Can you work these out from the model? Positions are in its coordinate system, mm. Face numbers are marked on the shaded views. A direction names the side the tool comes from. Give positions to 0.01 mm unless a question says otherwise; leave off trailing zeros. Order: outer loops, then holes, each group sorted by start corner. A loop starts at its lowest first (then second) coordinate and runs counter-clockwise, first axis right, second up. Notation, with made-up numbers: (63, 44.5) -> (70, 44.5) arc R34 cw to (70, 81.5) -> close; hole circle Ø7 at (70, 57). An arc over 180 degrees is marked (long way). Answer as a JSON object with one key per item and string values.
```python
from build123d import *

# Parameters (mm, degrees)
SKETCH1_R           = 110
BOSS_EXTRUDE1_DEPTH = 12
SKETCH2_R           = 110
BOSS_EXTRUDE2_DEPTH = 55
SKETCH3_W           = 100
SKETCH3_H           = 100
BOSS_EXTRUDE3_DEPTH = 80
SKETCH4_R           = 30
BOSS_EXTRUDE4_DEPTH = 20
BOSS_EXTRUDE4_TAPER = 18
SHELL1_T            = -1
SKETCH6_W           = 98
SKETCH6_H           = 6.826689401
BOSS_EXTRUDE5_DEPTH = 100
SKETCH7_W           = 98
SKETCH7_H           = 74.173310599
BOSS_EXTRUDE6_DEPTH = 15
SKETCH8_W           = 98
SKETCH8_H           = 4.922598218
BOSS_EXTRUDE7_DEPTH = 83


with BuildPart() as part:
    # Sketch1 → Boss-Extrude1 (new body)
    with BuildSketch(Plane(origin=(0, 0, 0), x_dir=(1, 0, 0), z_dir=(0, 1, 0))):
        with Locations(Location((0, 0, 0), (0, 0, 270))):
            Circle(SKETCH1_R)
        with BuildLine():
            Line((-4.5, 8.309783391), (-4.5, 23.309783391))
            Line((-4.5, 23.309783391), (4.5, 23.309783391))
            Line((4.5, 23.309783391), (4.5, 8.309783391))
            ThreePointArc((4.5, 8.309783391), (9.45, 0), (4.5, -8.309783391))
            Line((4.5, -8.309783391), (4.5, -23.309783391))
            Line((4.5, -23.309783391), (-4.5, -23.309783391))
            Line((-4.5, -23.309783391), (-4.5, -8.309783391))
            ThreePointArc((-4.5, -8.309783391), (-9.45, 0), (-4.5, 8.309783391))
        make_face(mode=Mode.SUBTRACT)
    extrude(amount=BOSS_EXTRUDE1_DEPTH)

    # Sketch2 → Boss-Extrude2 (add)
    with BuildSketch(Plane(origin=(0, 12, 0), x_dir=(1, 0, 0), z_dir=(0, 1, 0))):
        with Locations(Location((0, 0, 0), (0, 0, 270))):
            Circle(SKETCH2_R)
    extrude(amount=BOSS_EXTRUDE2_DEPTH)

    # Sketch3 → Boss-Extrude3 (add)
    with BuildSketch(Plane(origin=(0, 67, 0), x_dir=(1, 0, 0), z_dir=(0, 1, 0))):
        Rectangle(SKETCH3_W, SKETCH3_H)
    extrude(amount=BOSS_EXTRUDE3_DEPTH)

    # Sketch4 → Boss-Extrude4 (add)
    with BuildSketch(Plane.XY.offset(50)):
        with Locations((0, 107)):
            Circle(SKETCH4_R)
    extrude(amount=BOSS_EXTRUDE4_DEPTH, taper=BOSS_EXTRUDE4_TAPER)

    # Shell1
    shell1_openings = [part.faces().sort_by_distance(p)[0] for p in [
        (0, 147, 0),
    ]]
    offset(amount=SHELL1_T, openings=shell1_openings, kind=Kind.INTERSECTION)

    # Sketch6 → Boss-Extrude5 (add)
    with BuildSketch(Plane.XY.offset(-49)):
        with Locations((0, 69.413344701)):
            Rectangle(SKETCH6_W, SKETCH6_H)
    extrude(amount=BOSS_EXTRUDE5_DEPTH)

    # Sketch7 → Boss-Extrude6 (add)
    with BuildSketch(Plane.XY.offset(-49)):
        with Locations((0, 109.913344701)):
            Rectangle(SKETCH7_W, SKETCH7_H)
    extrude(amount=BOSS_EXTRUDE6_DEPTH)

    # Sketch8 → Boss-Extrude7 (add)
    with BuildSketch(Plane.XY.offset(-34)):
        with Locations((0, 144.538700891)):
            Rectangle(SKETCH8_W, SKETCH8_H)
    extrude(amount=BOSS_EXTRUDE7_DEPTH)


solid = part.part
```
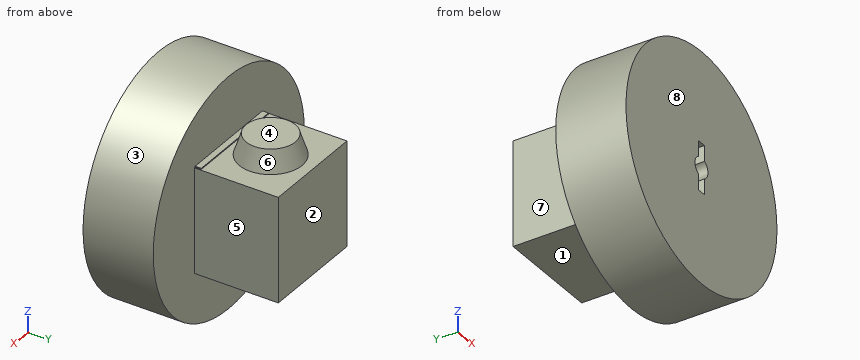
1. Will these pins go through, and if not, where does the flat tip stop? pin 1 Ø1.5 at (x, z) = (52, 52.5) entering from +Y; pin 2 Ø6 at (y, z) = (8, -17.5) entering from +X; pin 3 Ø23 at (x, y) = (-8.5, 106) entering from -Z; pin 4 Ø25 at (x, z) = (22, 22) entering from -Y.
Worked answers:
{"pin 1": "y = 67", "pin 2": "x = 109.04", "pin 3": "z = -50", "pin 4": "y = 0"}
2. Please list where these lines run through material, in increasing order: L1, parallel to Y at x = 48, z = -9.5; L2, parallel to Z at x = -45.5, y = 82; L3, parallel to Y at x = -87, z = -4.5.
Worked answers:
{"L1": "0 to 1, 66 to 72.83, 142.08 to 147", "L2": "-50 to -34, 49 to 50", "L3": "0 to 1, 66 to 67"}
3. If we section it at B-B on x = 0: Count the separate pieces of the cut face and the enclosed holes in it, then the cut area to 3 significant figures.
Worked answers:
{"separate pieces": "1", "enclosed holes": "2", "area": "2,880 mm²"}
4. If we section it at A-A on z = 0: Please give me the cut outline in (x, y), then the cut area to 3 significant figures.
Worked answers:
{"outline": "(-110, 0) -> (-9.45, 0) -> (-9.45, 12) -> (9.45, 12) -> (9.45, 0) -> (110, 0) -> (110, 67) -> (50, 67) -> (50, 147) -> (-50, 147) -> (-50, 67) -> (-110, 67) -> close; hole (-109, 1) -> (-10.45, 1) -> (-10.45, 13) -> (10.45, 13) -> (10.45, 1) -> (109, 1) -> (109, 66) -> (-109, 66) -> close; hole (-49, 72.83) -> (49, 72.83) -> (49, 142.08) -> (-49, 142.08) -> close", "area": "1,810 mm²"}
5. If we section it at C-C on y = 107: Please give me the cut outline in (x, z), then the cut area to 3 significant figures.
Worked answers:
{"outline": "(-50, -50) -> (50, -50) -> (50, 50) -> (30, 50) -> (23.5, 70) -> (-23.5, 70) -> (-30, 50) -> (-50, 50) -> close; hole (-49, -34) -> (49, -34) -> (49, 49) -> (29.27, 49) -> (22.78, 69) -> (-22.78, 69) -> (-29.27, 49) -> (-49, 49) -> close", "area": "1,900 mm²"}
6. For the marked faces 1, 2, 3, 4 and 5, which set-ups out of +Z, -Z, +X, -X, +Y, -Y let a thin tool reach every point of the face, with its end or its side?
Worked answers:
{"face 1": "-Z, +X, -X, +Y", "face 2": "+Z, -Z, +X, -X, +Y", "face 3": "+Y, -Y", "face 4": "+Z, +X, -X, +Y", "face 5": "+Z, -Z, +X, +Y"}
7. If we section it at D-D on z = -94: Please give me the cut outline in (x, y).
Worked answers:
{"outline": "(-57.13, 0) -> (57.13, 0) -> (57.13, 67) -> (-57.13, 67) -> close; hole (-55.18, 1) -> (55.18, 1) -> (55.18, 66) -> (-55.18, 66) -> close"}
8. If we mould it in two halves opening along Y, with no side actions, what happens to the marked faces 6, 7 and 8? For each: +Y half, -Y half, draft (parallel to the pull), parting line (faces both ways), or undercut.
Worked answers:
{"face 6": "undercut", "face 7": "draft", "face 8": "-Y half"}
